Source: CAD feature listing. Evaluate the final solid. Frame: model axes, mm. A direction names the side the tool comes from. Give positions to 0.01 mm unless a question says otherwise; leave off trailing zeros. Loops run counter-clockwise (first coordinate to the right, second up) from the corner with the lowest first, then second, coordinate; pieces in that order, holes last.
from build123d import *

# Parameters (mm, degrees)
SZKIC1_R                    = 2.9
DODANIE_WYCI_GNI_CIE1_DEPTH = 7.8
WYTNIJ_WYCI_GNI_CIE1_DEPTH  = 5
SZKIC3_R                    = 2.5
DODANIE_WYCI_GNI_CIE2_DEPTH = 51.7


with BuildPart() as part:
    # Szkic1 → Dodanie-wyciągnięcie1 (new body)
    with BuildSketch(Plane.XY):
        Circle(SZKIC1_R)
    extrude(amount=DODANIE_WYCI_GNI_CIE1_DEPTH)

    # Szkic2 → Wytnij-wyciągnięcie1 (cut)
    with BuildSketch(Plane.XY.offset(7.8)):
        Polygon((0, -0.45), (2.86487347, -0.45), (2.86487347, -2.9), (-2.9, -2.9), (-2.9, -0.45), align=None)
        Polygon((0, 0.45), (2.86487347, 0.45), (2.86487347, 2.9), (-3.305563266, 2.9), (-3.305563266, 0.45), align=None)
    extrude(amount=-WYTNIJ_WYCI_GNI_CIE1_DEPTH, mode=Mode.SUBTRACT)

    # Szkic3 → Dodanie-wyciągnięcie2 (add)
    with BuildSketch(Plane(origin=(0, 0, 0), x_dir=(-1, 0, 0), z_dir=(0, 0, -1))):
        Circle(SZKIC3_R)
    extrude(amount=DODANIE_WYCI_GNI_CIE2_DEPTH)

    # Szkic7 → Otwór Ø3.5 (3.5)2 (revolve, cut)
    with BuildSketch(Plane(origin=(0, 0, -51.7), x_dir=(0, 1, 0), z_dir=(1, 0, 0))):
        Polygon((0, 0), (0, 18.051506083), (1.75, 17), (1.75, 0), align=None)
    revolve(axis=Axis((0, 0, -58.05), (0, 0, 1)), mode=Mode.SUBTRACT)


solid = part.part
1) Reachability of faces 1 (the flat face through (2, -1, -51.7)), 2 (the cylindrical face through (0.54, -2.44, -25.49)), 3 (the flat face through (0, -1, 2.8)), 4 (the flat face through (0, 1, 2.8)) from +Z, -Z, +X, -X, +Y, -Y: full face, straight path, thin tool, end or side. Return the list, or none.
Checks:
face 1: -Z, +X, -X, +Y, -Y
face 2: -Z
face 3: +Z, +X, -X, -Y
face 4: +Z, +X, -X, +Y
2) Cut plane A-A (z = -1.5). Return loops of the section in (x, y).
Checks:
outline: circle Ø5 at (0, 0)
3) Pull-direction query (X, two-part tool) for faces 5 (the flat face through (0, -0.45, 5)), 6 (the cylindrical face through (-2.9, 0.1, 2.1)), 7 (the conical face through (0.297, -0.066, -33.831)); classes: released by +X, released by -X, zero draft, split by the parting line, or undercut.
Checks:
face 5: zero draft
face 6: split by the parting line
face 7: undercut
4) Ray query, probe 1 along Y at (x, z) = (0, -39); probe 2 along Z at (x, y) = (-1.7, 0.8); probe 3 along X at (y, z) = (-0.1, -22). Return the intervals inside material, ascending.
Checks:
probe 1: y = -2.5 to -1.75, 1.75 to 2.5
probe 2: z = -51.7 to 2.8
probe 3: x = -2.5 to 2.5
5) Contact query for flat-ended pins moving along their axis: P1, Ø2.5, axis at x = 0, y = -2, coming from the +Z side; P2, Ø3, axis at y = 1, z = -3, coming from the -X side; P3, Ø1.5, axis at y = 2, z = -29.5, coming from the +X side. Output: stop coordinate, or through.
Checks:
P1: stops at z = 2.8
P2: stops at x = -2.5
P3: stops at x = 2.17
